```python
from build123d import *

# Parameters (mm, degrees)
F1_DEPTH  = 6.35
F2_W      = 25.4
F2_H      = 12.7
F3_DEPTH  = 57.15
F5_DEPTH  = 12.701
F6_DEPTH  = 12.7
F7_R      = 6.35
F8_DEPTH  = 25.401
F9_W      = 12.7
F9_H      = 12.7
F10_DEPTH = 25.4
F12_DEPTH = 12.701
F13_R     = 3.175
F14_DEPTH = 6.351


with BuildPart() as f1:
    # F0 (on Top) → F1 (new body)
    with BuildSketch(Plane.XY):
        with BuildLine():
            Line((0, 31.75), (-50.8, 31.75))
            Line((-50.8, 31.75), (-50.8, 12.7))
            ThreePointArc((-50.8, 12.7), (-46.87018, 3.92982), (-38.1, 0))
            Line((-38.1, 0), (-12.7, 0))
            ThreePointArc((-12.7, 0), (-3.92982, 3.92982), (0, 12.7))
            Line((0, 12.7), (0, 31.75))
        make_face()
    extrude(amount=F1_DEPTH)

    # F2 (on face) → F3 (join)
    with BuildSketch(Plane.XY.offset(6.35)):
        with Locations((-25.4, 25.4)):
            Rectangle(F2_W, F2_H)
    extrude(amount=F3_DEPTH)

    # F4 (on face) → F5 (cut, through all)
    with BuildSketch(Plane.XZ.offset(-19.05)):
        with BuildLine():
            ThreePointArc((-25.4, 63.5), (-16.419744, 59.780256), (-12.7, 50.8))
            Line((-12.7, 50.8), (-12.7, 63.5))
            Line((-12.7, 63.5), (-25.4, 63.5))
        make_face()
        with BuildLine():
            ThreePointArc((-38.1, 50.8), (-34.380256, 59.780256), (-25.4, 63.5))
            Line((-25.4, 63.5), (-38.1, 63.5))
            Line((-38.1, 63.5), (-38.1, 50.8))
        make_face()
    extrude(amount=-F5_DEPTH, mode=Mode.SUBTRACT)

    # F4 (on face) → F6 (join)
    with BuildSketch(Plane.XZ.offset(-19.05)):
        with BuildLine():
            ThreePointArc((-38.1, 50.8), (-25.4, 38.1), (-12.7, 50.8))
            ThreePointArc((-12.7, 50.8), (-16.419744, 59.780256), (-25.4, 63.5))
            ThreePointArc((-25.4, 63.5), (-34.380256, 59.780256), (-38.1, 50.8))
        make_face()
    extrude(amount=F6_DEPTH)

    # F7 (on face) → F8 (cut, through all)
    with BuildSketch(Plane.XZ.offset(-6.35)):
        with Locations((-25.4, 50.8)):
            Circle(F7_R)
    extrude(amount=-F8_DEPTH, mode=Mode.SUBTRACT)

    # F9 (on face) → F10 (join)
    with BuildSketch(Plane.XY.offset(6.35)):
        with Locations((-44.45, 25.4)):
            Rectangle(F9_W, F9_H)
        with Locations((-6.35, 25.4)):
            Rectangle(F9_W, F9_H)
    extrude(amount=F10_DEPTH)

    # F11 (on face) → F12 (cut, through all)
    with BuildSketch(Plane.XZ.offset(-19.05)):
        with BuildLine():
            Line((-38.1, 19.05), (-38.1, 31.75))
            Line((-38.1, 31.75), (-50.8, 31.75))
            Line((-50.8, 31.75), (-50.8, 6.35))
            ThreePointArc((-50.8, 6.35), (-41.819744, 10.069744), (-38.1, 19.05))
        make_face()
        with BuildLine():
            Line((0, 31.75), (-12.7, 31.75))
            Line((-12.7, 31.75), (-12.7, 19.05))
            ThreePointArc((-12.7, 19.05), (-8.980256, 10.069744), (0, 6.35))
            Line((0, 6.35), (0, 31.75))
        make_face()
    extrude(amount=-F12_DEPTH, mode=Mode.SUBTRACT)

    # F13 (on face) → F14 (cut, through all)
    with BuildSketch(Plane.XY.offset(6.35)):
        with Locations((-41.275, 9.525)):
            Circle(F13_R)
        with Locations((-9.525, 9.525)):
            Circle(F13_R)
    extrude(amount=-F14_DEPTH, mode=Mode.SUBTRACT)


solid = f1.part
```
Here's how the part is built. I have some questions about the finished solid (model axes, mm). A direction names the side the tool comes from. Round coordinates to 2 decimals unless told otherwise and drop trailing zeros. Write each loop counter-clockwise with the first axis right and the second up, starting at its lowest first coordinate (ties: lowest second). Pieces come first, ordered by that corner, then holes.
Q1. Will these pins go through, and if not, where does the flat tip stop? P1, Ø4, axis at y = 28, z = 35, coming from the -X side; P2, Ø2, axis at x = -11.5, z = 56.5, coming from the -Y side; P3, Ø10, axis at y = 27, z = 39, coming from the +X side; P4, Ø12.5, axis at x = -19.5, z = 50.5, coming from the -Y side.
Q2. If we section it at A-A on y = 17.5: Write out the boundary of the cut face in (x, z), plus the area to 3 significant figures.
Q3. Which directions (+Z, -Z, +X, -X, +Y, -Y) give clear straight access to the entire face, cutting with the end or side of a thin tool? Please do faces 5 (the flat face through (-12.7, 25, 35)), 6 (the flat face through (-26, 10, 6.35)), 7 (the flat face through (-23, 6.35, 57)), 8 (the flat face through (-38.1, 25, 35)).
Q4. If we section it at D-D on z = 35.5: Write out the boundary of the cut face in (x, y), plus the area to 3 significant figures.
Q5. If we section it at B-B on x = -39: Write out the boundary of the cut face in (y, z), plus the area to 3 significant figures.
Q6. Please list where these lines run through material, in increasing order: probe 1 along Z at (x, y) = (-25, 17); probe 2 along Z at (x, y) = (-25, 26); probe 3 along X at (y, z) = (9, 4.5).
Q7. If we section it at C-C on y = 26: Write out the boundary of the cut face in (x, z), plus the area to 3 significant figures.
Q8. If we mould it in two halves opening along Z, with no side actions, what happens to faces 1 (the cylindrical face through (-26.2, 18.9, 57.1)), 2 (the cylindrical face through (-41.92, 25.31, 9.97)), 3 (the flat face through (-26, 19.05, 23)), 4 (the cylindrical face through (-44.447, 9.665, 3.219))? For each: +Z half, -Z half, draft (parallel to the pull), parting line (faces both ways), or undercut.
Answer below:
1. P1: stops at x = -38.1
1. P2: passes through
1. P3: stops at x = -12.7
1. P4: stops at y = 6.35
2. outline: (-50.8, 0) - (0, 0) - (0, 6.35) - (-50.8, 6.35) - close; circle Ø25.4 at (-25.4, 50.8); hole circle Ø12.7 at (-25.4, 50.8)
2. area: 703 mm2
3. face 5: +Z, +X, +Y, -Y
3. face 6: +X, -X, -Y
3. face 7: +Z, +X, -X, -Y
3. face 8: +Z, -X, +Y, -Y
4. outline: (-38.1, 19.05) - (-12.7, 19.05) - (-12.7, 31.75) - (-38.1, 31.75) - close
4. area: 323 mm2
5. outline: (0.08, 0) - (7.31, 0) - (7.31, 6.35) - (0.08, 6.35) - close; (11.74, 0) - (31.75, 0) - (31.75, 14.35) - (19.05, 14.35) - (19.05, 6.35) - (11.74, 6.35) - close
5. area: 275 mm2
6. probe 1: z = 0 to 6.35, 38.11 to 44.46, 57.14 to 63.49
6. probe 2: z = 0 to 44.46, 57.14 to 63.49
6. probe 3: x = -50.06 to -44.41, -38.14 to -12.66, -6.39 to -0.74
7. outline: (-50.8, 0) - (0, 0) - (0, 6.35) arc R12.7 cw to (-12.7, 19.05) - (-12.7, 50.8) arc R12.7 ccw to (-38.1, 50.8) - (-38.1, 19.05) arc R12.7 cw to (-50.8, 6.35) - close; hole circle Ø12.7 at (-25.4, 50.8)
7. area: 1,650 mm2
8. face 1: undercut
8. face 2: +Z half
8. face 3: undercut
8. face 4: draft
